Input: dimensioned drawing with shaded views. Units: mm. Origin: part minimum x, y, z. A direction names the side the tool comes from. Coordinates: 2 decimals unless noted, no trailing zeros. Order: outer loops, then holes, each group sorted by start corner. A loop starts at its lowest first (then second) coordinate and runs counter-clockwise, first axis right, second up. Notation, with made-up numbers: (25, -27) - (45, -27) arc R16 cw to (45, -12) - close; hole circle Ø6 at (-19, -14). An arc over 180 degrees is marked (long way). Answer as CSV lines item,"result". Start each with the question number.
Item 1: Material intervals for line 1 along X through (y, z) = (3.75, 12); line 2 along Z through (x, y) = (37.5, 10); line 3 along Z through (x, y) = (15, 1.5), sorted ascending.
Item 2: Section A-A (x = 78.5). Output: boundary loops of the cut face in (y, z), and give its area (3 significant figures).
Item 3: Section B-B (y = 7). Output: boundary loops of the cut face in (x, z), and give its area (3 significant figures).
Item 4: Access query for the marked faces 1, 2 and 3. Directions: +Z, -Z, +X, -X, +Y, -Y. A direction counts if a zero-diameter tool reaches every point of the face in a straight line with its end or side. Return the directions, or none.
Item 5: Section C-C (z = 97). Output: boundary loops of the cut face in (x, y).
Item 6: First-contact query: pin 1 (4 mm diameter, centred on x = 10, y = 4.5, fed in from -Z); pin 2 (4 mm diameter, centred on x = 49, y = 11, fed in from +Z); pin 3 (6 mm diameter, centred on y = 9, z = 109, fed in from +X). Flat tips, straight axial feed; report the tip coordinate or a pass-through.
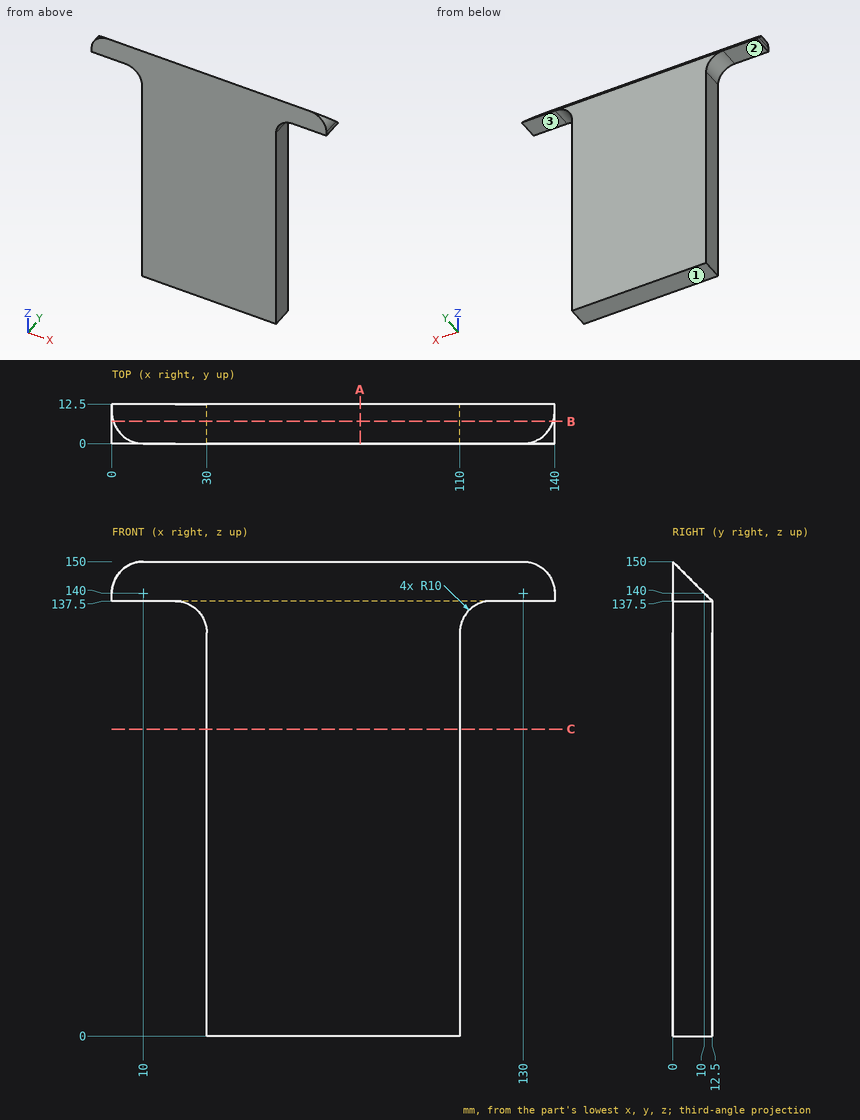
Determined:
1,line 1,"x = 30 to 110"
1,line 2,"z = 0 to 140"
1,line 3,"z = 137.5 to 148.5"
2,outline,"(0, 0) - (12.5, 0) - (12.5, 137.5) - (0, 150) - close"
2,area,"1,800 mm^2"
3,outline,"(0, 137.5) - (20, 137.5) arc R10 cw to (30, 127.5) - (30, 0) - (110, 0) - (110, 127.5) arc R10 cw to (120, 137.5) - (140, 137.5) - (140, 140) arc R10 ccw to (139.54, 143) - (0.46, 143) arc R10 ccw to (0, 140) - close"
3,area,"11,800 mm^2"
4,face 1,"-Z, +X, -X, +Y, -Y"
4,face 2,"-Z, -X, +Y, -Y"
4,face 3,"-Z, +X, +Y, -Y"
5,outline,"(30, 0) - (110, 0) - (110, 12.5) - (30, 12.5) - close"
6,pin 1,"stops at z = 137.5"
6,pin 2,"stops at z = 141"
6,pin 3,"stops at x = 110"
